The listing builds one solid part. Answer for the finished solid, in the listing's coordinates (mm). A direction names the side the tool comes from. Give positions to 0.01 mm unless a question says otherwise; leave off trailing zeros. Order: outer loops, then holes, each group sorted by start corner. A loop starts at its lowest first (then second) coordinate and runs counter-clockwise, first axis right, second up. Notation, with made-up numbers: (19, -40) -> (73, -40) arc R28 cw to (73, -8) -> close; hole circle Ø4 at (57.25, -3.5). An arc over 180 degrees is marked (long way). Write item = value, one per line. Start each with the question number.
```python
from build123d import *

# Parameters (mm, degrees)
F1_DEPTH = 6
F2_W     = 22
F2_H     = 3
F3_DEPTH = 6


with BuildPart() as f1:
    # F0 (on Top) → F1 (new body)
    with BuildSketch(Plane.XY):
        with BuildLine():
            Line((-28, 0), (0, 0))
            Line((0, 0), (0, 10))
            ThreePointArc((0, 10), (8.5, 27.613915), (0, 45.22783))
            Line((0, 45.22783), (0, 55.272548))
            Line((0, 55.272548), (-28, 55.272548))
            Line((-28, 55.272548), (-28, 45.22783))
            ThreePointArc((-28, 45.22783), (-36.5, 27.613915), (-28, 10))
            Line((-28, 10), (-28, 0))
        make_face()
    extrude(amount=F1_DEPTH)

    # F2 (on face) → F3 (cut, through all)
    with BuildSketch(Plane.XY.offset(6)):
        with Locations((-14, 53.772548)):
            Rectangle(F2_W, F2_H)
        with Locations((-14, 1.5)):
            Rectangle(F2_W, F2_H)
    extrude(amount=-F3_DEPTH, mode=Mode.SUBTRACT)


solid = f1.part
```
Item 1: Which of the six approach directions +Z, -Z, +X, -X, +Y, -Y give full straight-line access (tool end or side, diameter ignored) to faces 1 (the flat face through (0, 50, 3)), 2 (the flat face through (-28, 50, 3)), 3 (the flat face through (-14, 3, 3)), 4 (the flat face through (-3, 54, 3))?
Item 2: Flat-ended cylindrical pins translate along their axes: pin 1 (2.5 mm diameter, centred on y = 1.5, z = 2.5, fed in from -X); pin 2 (0.9 mm diameter, centred on y = 53, z = 2.5, fed in from +X); pin 3 (1 mm diameter, centred on x = -30, z = 4, fed in from +Y). Find the tip coordinate at first contact, or state that the pin passes through.
Item 3: The mould has two halves that part along X. Classify faces 5 (the flat face through (-26, 55.273, 3)), 6 (the cylindrical face through (8.5, 27.33, 2.96)), 7 (the flat face through (-14, 52.273, 3)): +X half, -X half, draft (parallel to the pull), parting line (faces both ways), or undercut.
Item 4: A cutting plane is placed at B-B, the plane y = 48. Write down the section's boundary in (x, z), plus the area to 3 significant figures.
Item 5: A cutting plane is placed at A-A, the plane z = 2.35. Write down the section's boundary in (x, y).
Item 6: A cutting plane is placed at C-C, the plane x = -10. Write down the section's boundary in (y, z).
Item 7: Consider L1, parallel to Y at x = -13, z = 2.5; L2, parallel to X at y = 4, z = 5.2; L3, parallel to Y at x = -29, z = 5.6. Determine where each line is inside the solid, lowest interval first. Write a range as from..to.
Check values:
q1.face_1 = +Z, -Z, +X, +Y
q1.face_2 = +Z, -Z, -X, +Y
q1.face_3 = +Z, -Z, -Y
q1.face_4 = +Z, -Z, +Y
q2.pin_1 = -28
q2.pin_2 = 0
q2.pin_3 = 43.92
q3.face_5 = draft
q3.face_6 = +X half
q3.face_7 = undercut
q4.outline = (-28, 0) -> (0, 0) -> (0, 6) -> (-28, 6) -> close
q4.area = 168 mm^2
q5.outline = (-28, 0) -> (-25, 0) -> (-25, 3) -> (-3, 3) -> (-3, 0) -> (0, 0) -> (0, 10) arc R22.5 ccw to (0, 45.23) -> (0, 55.27) -> (-3, 55.27) -> (-3, 52.27) -> (-25, 52.27) -> (-25, 55.27) -> (-28, 55.27) -> (-28, 45.23) arc R22.5 ccw to (-28, 10) -> close
q6.outline = (3, 0) -> (52.27, 0) -> (52.27, 6) -> (3, 6) -> close
q7.L1 = 3..52.27
q7.L2 = -28..0
q7.L3 = 10.84..44.38
